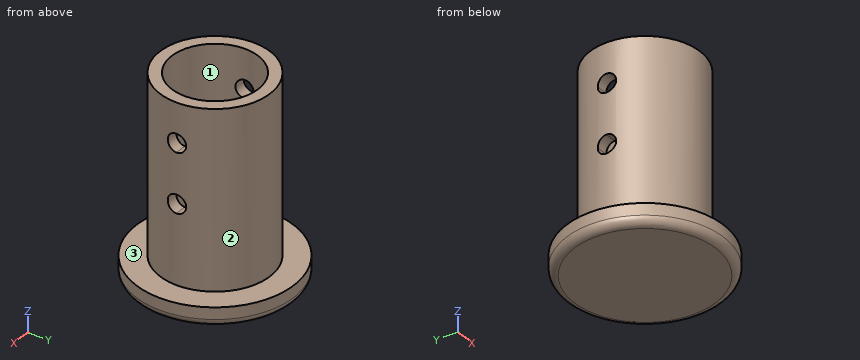
```python
from build123d import *

# Parameters (mm, degrees)
F0_R          = 14
F0_R_2        = 11
F1_DEPTH      = 50
F0_R_3        = 20
F2_DEPTH      = 5
F3_DEPTH      = 5
F4_R          = 2
F6_DEPTH      = 20.0010001
F6_DEPTH_BACK = 25


with BuildPart() as f1:
    # F0 (on Top) → F1 (new body)
    with BuildSketch(Plane.XY):
        Circle(F0_R)
        Circle(F0_R_2, mode=Mode.SUBTRACT)
    extrude(amount=F1_DEPTH)

    # F0 (on Top) → F2 (join)
    with BuildSketch(Plane.XY):
        Circle(F0_R_3)
        Circle(F0_R, mode=Mode.SUBTRACT)
    extrude(amount=F2_DEPTH)

    # F0 (on Top) → F3 (join)
    with BuildSketch(Plane.XY):
        Circle(F0_R_2)
    extrude(amount=F3_DEPTH)

    # F4
    f4_edges = [f1.edges().sort_by_distance(p)[0] for p in [
        (-20, 0, 0),
    ]]
    fillet(f4_edges, radius=F4_R)

    # F5 (on Right) → F6 (cut, two sides)
    with BuildSketch(Plane.YZ) as f6_sk:
        with BuildLine():
            ThreePointArc((2.325, 40), (-1.6440232663, 41.6440232663), (0, 37.675))
            ThreePointArc((0, 37.675), (1.6440232663, 38.3559767337), (2.325, 40))
        make_face()
        with BuildLine():
            Line((0, 25), (0, 22.675))
            ThreePointArc((0, 22.675), (1.6440232663, 23.3559767337), (2.325, 25))
            ThreePointArc((2.325, 25), (1.6440232663, 26.6440232663), (0, 27.325))
            Line((0, 27.325), (0, 25))
        make_face()
        with BuildLine():
            ThreePointArc((0, 27.325), (-2.325, 25), (0, 22.675))
            Line((0, 22.675), (0, 25))
            Line((0, 25), (0, 27.325))
        make_face()
    extrude(amount=-F6_DEPTH, mode=Mode.SUBTRACT)
    extrude(f6_sk.sketch, amount=F6_DEPTH_BACK, mode=Mode.SUBTRACT)


solid = f1.part
```
Could you check a few things on this model? Use its own coordinates, in mm. Face numbers are marked on the shaded views. Give positions to 0.01 mm unless a question says otherwise; leave off trailing zeros. Loops run counter-clockwise (first coordinate to the right, second up) from the corner with the lowest first, then second, coordinate; pieces in that order, holes last. Notation, with made-up numbers: (31, 57) - (45, 57) arc R20 ccw to (45, 70) - close; hole circle Ø7 at (-35, -6). An arc over 180 degrees is marked (long way). Use one line per item in the form item = value.
1. Thinking about a two-plate mould opening in Y: for the marked faces 1, 2 and 3, which applies, released by +Y, released by -Y, zero draft, split by the parting line, or undercut?
Response values:
face_1 = undercut
face_2 = split by the parting line
face_3 = zero draft
2. I need wall thicknesses on probe 1 along X at (y, z) = (0, 20); probe 2 along Z at (x, y) = (5, -17). Which ranges of each line are inside material? Lowest first, please.
Response values:
probe_1 = -14 to -11, 11 to 14
probe_2 = 0 to 5
3. I want a section at C-C (z = 3.5). Please give me the cut outline in (x, y).
Response values:
outline = circle Ø40 at (0, 0)
4. I'm going to push flat-ended pins straight in: pin 1 Ø7.5 at (y, z) = (0, 40) entering from -X; pin 2 Ø1 at (y, z) = (1.5, 30.5) entering from +X; pin 3 Ø4 at (y, z) = (0, 40) entering from +X; pin 4 Ø10 at (x, z) = (-10.5, 35.5) entering from -Y. Where does each tip first touch, or does it pass through?
Response values:
pin_1 = -14
pin_2 = 13.96
pin_3 = through
pin_4 = -12.87
5. I want a section at A-A (z = 26). Please give me the cut outline in (x, y).
Response values:
outline = (-13.84, -2.1) arc R14 ccw to (13.84, -2.1) - (10.8, -2.1) arc R11 cw to (-10.8, -2.1) - close; (-13.84, 2.1) - (-10.8, 2.1) arc R11 cw to (10.8, 2.1) - (13.84, 2.1) arc R14 ccw to start
6. I want a section at B-B (x = 0). Please give me the cut outline in (y, z), and give its area (3 significant figures).
Response values:
outline = (-20, 2) arc R2 ccw to (-18, 0) - (18, 0) arc R2 ccw to (20, 2) - (20, 5) - (14, 5) - (14, 50) - (11, 50) - (11, 5) - (-11, 5) - (-11, 50) - (-14, 50) - (-14, 5) - (-20, 5) - close
area = 468 mm²
